from build123d import *

# Parameters (mm, degrees)
SKETCH3_R           = 1.05
BOSS_EXTRUDE1_DEPTH = 1


with BuildPart() as part:
    # Sketch3 → Boss-Extrude1 (new body)
    with BuildSketch(Plane.XY):
        with BuildLine():
            Line((0, 14.052488348), (55, 14.052488348))
            ThreePointArc((55, 14.052488348), (58.535533906, 12.588022254), (60, 9.052488348))
            Line((60, 9.052488348), (60, -8.947511652))
            ThreePointArc((60, -8.947511652), (58.535533906, -12.483045558), (55, -13.947511652))
            Line((55, -13.947511652), (0, -13.947511652))
            Line((0, -13.947511652), (-55, -13.947511652))
            ThreePointArc((-55, -13.947511652), (-58.535533906, -12.483045558), (-60, -8.947511652))
            Line((-60, -8.947511652), (-60, 9.052488348))
            ThreePointArc((-60, 9.052488348), (-58.535533906, 12.588022254), (-55, 14.052488348))
            Line((-55, 14.052488348), (0, 14.052488348))
        make_face()
        with Locations((-56.327907587, 10.548035553)):
            Circle(SKETCH3_R, mode=Mode.SUBTRACT)
        with Locations((56.327907587, 10.548035553)):
            Circle(SKETCH3_R, mode=Mode.SUBTRACT)
        with Locations((-14.5, -10.947511652)):
            Circle(SKETCH3_R, mode=Mode.SUBTRACT)
        with Locations((14.5, -10.947511652)):
            Circle(SKETCH3_R, mode=Mode.SUBTRACT)
    extrude(amount=BOSS_EXTRUDE1_DEPTH)


solid = part.part
The model under review builds one solid part; all positions refer to its coordinate system, in mm. Give positions to 0.01 mm unless a question says otherwise; leave off trailing zeros. Order: outer loops, then holes, each group sorted by start corner. A loop starts at its lowest first (then second) coordinate and runs counter-clockwise, first axis right, second up. Notation, with made-up numbers: (50.5, 59.25) -> (82.5, 59.25) arc R27 ccw to (82.5, 90.25) -> close; hole circle Ø1 at (-9, 39.25). An arc over 180 degrees is marked (long way). Write item = value, one per line. Start each with the question number.
(1) For pin 1 Ø4 at (x, y) = (39, -7) entering from -Z, flat-tipped, find the tip position at first contact; note if it passes through.
(2) For L1, parallel to X at y = 11, z = 0.45; L2, parallel to X at y = 10.75, z = 0.75; L3, parallel to Y at x = 14.5, z = 0.85, list the stretches that pass through material, from the lowest coordinate up. Write a range as from..to.
(3) Draft analysis for pull direction Y (two halves, no side actions). For faces 1 (the cylindrical face through (-58.5, -12.52, 0.49)), 2 (the flat face through (1, 0, 1)), 3 (the cylindrical face through (13.45, -10.9, 0.49)), state which applies: +Y half, -Y half, draft (parallel to the pull), parting line (faces both ways), or undercut.
(4) Take a section at A-A (x = 14.5). Write out the cut boundary in (y, z).
Returned:
q1.pin_1 = 0
q2.L1 = -59.61..-57.28, -55.38..55.38, 57.28..59.61
q2.L2 = -59.7..-57.36, -55.3..55.3, 57.36..59.7
q2.L3 = -13.95..-12, -9.9..14.05
q3.face_1 = -Y half
q3.face_2 = draft
q3.face_3 = undercut
q4.outline = (-13.95, 0) -> (-12, 0) -> (-12, 1) -> (-13.95, 1) -> close; (-9.9, 0) -> (14.05, 0) -> (14.05, 1) -> (-9.9, 1) -> close
